Here's how the part is built. I have some questions about the finished solid (model axes, mm). A direction names the side the tool comes from. Coordinates: 2 decimals unless noted, no trailing zeros. Loops run counter-clockwise (first coordinate to the right, second up) from the corner with the lowest first, then second, coordinate; pieces in that order, holes last. Notation, with made-up numbers: M 57,63.25 L 74,63.25 A17 ccw 74,85.25 Z; hole C 87,34.25 d6. An arc over 180 degrees is marked long. Use one line per item in the form item = value. Start each with the question number.
(1) Thinking about a two-plate mould opening in Y: for faces 1 (the flat face through (16, 0, -6)), 2 (the flat face through (1, 10, -6)), 3 (the flat face through (1, 25, -6)), which applies, +Y half, -Y half, draft (parallel to the pull), parting line (faces both ways), or undercut?
(2) Imagine slicing it at D-D, the plane y = -20. Please give me the cut outline in (x, z).
(3) Will these pins go through, and if not, where does the flat tip stop? P1, Ø1, axis at x = 26, y = -4.5, coming from the -Z side; P2, Ø12, axis at x = 0.5, y = -15, coming from the +Z side; P3, Ø1.5, axis at x = 14.5, z = -10.5, coming from the +Y side.
(4) Imagine slicing it at C-C, the plane z = -6. Please give me the cut outline in (x, y), and give its area (3 significant figures).
(5) On a 3-axis mill with a long thin cutter (end or side, diameter ignored), from which of +Z, -Z, +X, -X, +Y, -Y can I reach the whole of each face in a straight line? I mean faces 4 (the flat face through (16, 5, -6)), 5 (the flat face through (6, 20, -6)), 6 (the flat face through (23, -15, -6)). Say none if no direction works.
(6) Imagine slicing it at A-A, the plane y = 22. Please give me the cut outline in (x, z).
(7) Please list where these lines run through material, in increasing order: L1, parallel to X at y = 13.5, z = -10.75; L2, parallel to Y at x = 4, z = -1.5; L3, parallel to Y at x = 11, z = -0.25.
(8) Imagine slicing it at B-B, the plane z = -12.75. Please give me the cut outline in (x, y).
```python
from build123d import *
from build123d.topology import SkipClean

# Parameters (mm, degrees)
SKETCH_3_W          = 32
SKETCH_3_H          = 12
EXTRUDE_3_DEPTH     = 5
SKETCH_4_R          = 5
EXTRUDE_4_DEPTH     = 10
SKETCH_8_R          = 5
EXTRUDE_6_DEPTH     = 5
SKETCH_9_R          = 4.8
CUT_EXTRUDE_2_DEPTH = 0.5
EXTRUDE_START       = 5
SKETCH_36_R         = 5
SKETCH_36_R_2       = 4.98
EXTRUDE_11_DEPTH    = 5
SKETCH_46_W         = 32
SKETCH_46_H         = 12
EXTRUDE_12_DEPTH    = 20
SKETCH_47_W         = 4
SKETCH_47_H         = 25
EXTRUDE_13_DEPTH    = 12
SKETCH_48_W         = 4
SKETCH_48_H         = 25
EXTRUDE_14_DEPTH    = 12
CUT_EXTRUDE_START   = -12
CUT_EXTRUDE_5_DEPTH = 12
SKETCH_50_R         = 6
EXTRUDE_15_DEPTH    = 20
SKETCH_51_R         = 6
EXTRUDE_16_DEPTH    = 20
SKETCH_54_R         = 6
EXTRUDE_17_DEPTH    = 25
SKETCH_55_R         = 6
EXTRUDE_18_DEPTH    = 25
SKETCH_56_R         = 6
CUT_EXTRUDE_6_DEPTH = 10
SKETCH_57_R         = 2.5
EXTRUDE_19_DEPTH    = 10
SKETCH_58_R         = 6
SKETCH_58_R_2       = 2.5
CUT_EXTRUDE_8_DEPTH = 10
EXTRUDE_20_DEPTH    = 2.5
EXTRUDE_21_DEPTH    = 2.5


# Read off the part's stored shape, not the designer's step: the extrude step
with BuildPart() as part:
    # Sketch 3 → Extrude 3 (new body)
    with BuildSketch(Plane(origin=(0, 0, 0), x_dir=(1, 0, 0), z_dir=(0, 1, 0))):
        with Locations((16, 6)):
            Rectangle(SKETCH_3_W, SKETCH_3_H)
    extrude(amount=EXTRUDE_3_DEPTH)

    # Sketch 4 → Extrude 4 (add)
    with BuildSketch(Plane.XZ):
        with Locations(Location((6, -6, 0), (0, 0, 270))):
            Circle(SKETCH_4_R)
        with Locations(Location((26, -6, 0), (0, 0, 270))):
            Circle(SKETCH_4_R)
    extrude(amount=EXTRUDE_4_DEPTH)

    # Sketch 8 → Extrude 6 (add)
    with BuildSketch(Plane.XZ.offset(10)):
        with Locations(Location((6, -6, 0), (0, 0, 270))):
            Circle(SKETCH_8_R)
    extrude(amount=EXTRUDE_6_DEPTH)

    # Sketch 9 → Cut-Extrude 2 (cut)
    with BuildSketch(Plane.XZ.offset(15)):
        with Locations(Location((6, -6, 0), (0, 0, 270))):
            Circle(SKETCH_9_R)
    extrude(amount=-CUT_EXTRUDE_2_DEPTH, mode=Mode.SUBTRACT)



with BuildPart() as body_2:
    # Sketch 14 → Revolve 2 (revolve)
    with BuildSketch(Plane.XY.offset(-6), mode=Mode.PRIVATE) as revolve_2_sk:
        Polygon((1.021282046, -15), (1.021282046, -20), (1.221282046, -15), align=None)
    revolve(revolve_2_sk.sketch.rotate(Axis((6, -15, -6), (0, 1, 0)), 270), axis=Axis((6, -15, -6), (0, 1, 0)))


with BuildPart() as part_1:
    with SkipClean():  # the faces are left unmerged after this step: merging them gives an invalid solid
        add(part.part)

        add(body_2.part)  # Extrude 11 merges body 2
        # Sketch 36 → Extrude 11 (add)
        with BuildSketch(Plane(origin=(0, -20, 0), x_dir=(1, 0, 0), z_dir=(0, 1, 0)).offset(EXTRUDE_START)):
            with Locations(Location((6, 6, 0), (0, 0, 270))):
                Circle(SKETCH_36_R)
            with Locations(Location((6, 6, 0), (0, 0, 90))):
                Circle(SKETCH_36_R_2, mode=Mode.SUBTRACT)
        extrude(amount=-EXTRUDE_11_DEPTH)

    # Sketch 46 → Extrude 12 (add)
    with SkipClean():  # the faces are left unmerged after this step: merging them gives an invalid solid
        with BuildSketch(Plane(origin=(0, 5, 0), x_dir=(1, 0, 0), z_dir=(0, 1, 0))):
            with Locations((16, 6)):
                Rectangle(SKETCH_46_W, SKETCH_46_H)
        extrude(amount=EXTRUDE_12_DEPTH)

    # Sketch 47 → Extrude 13 (add)
    with SkipClean():  # the faces are left unmerged after this step: merging them gives an invalid solid
        with BuildSketch(Plane.XY):
            with Locations((-2, 12.5)):
                Rectangle(SKETCH_47_W, SKETCH_47_H)
        extrude(amount=-EXTRUDE_13_DEPTH)

    # Sketch 48 → Extrude 14 (add)
    with SkipClean():  # the faces are left unmerged after this step: merging them gives an invalid solid
        with BuildSketch(Plane.XY):
            with Locations((34, 12.5)):
                Rectangle(SKETCH_48_W, SKETCH_48_H)
        extrude(amount=-EXTRUDE_14_DEPTH)

    # Cut-Extrude 5 outline → Cut-Extrude 5 (cut)
    with SkipClean():  # the faces are left unmerged after this step: merging them gives an invalid solid
        with BuildSketch(Plane.XY.offset(CUT_EXTRUDE_START)):
            Polygon((26, 25), (6, 25), (6, 15), (1, 15), (1, 5), (31, 5), (31, 15), (26, 15), align=None)
        extrude(amount=CUT_EXTRUDE_5_DEPTH, mode=Mode.SUBTRACT)

    # Sketch 50 → Extrude 15 (add)
    with BuildSketch(Plane.XZ):
        with Locations(Location((6, -6, 0), (0, 0, 270))):
            Circle(SKETCH_50_R)
    extrude(amount=EXTRUDE_15_DEPTH)

    # Sketch 51 → Extrude 16 (add)
    with BuildSketch(Plane.XZ):
        with Locations(Location((26, -6, 0), (0, 0, 270))):
            Circle(SKETCH_51_R)
    extrude(amount=EXTRUDE_16_DEPTH)

    # Sketch 52 → Revolve 3 (revolve)
    with BuildSketch(Plane.XY.offset(-6), mode=Mode.PRIVATE) as revolve_3_sk:
        Polygon((0, -20), (0, -25), (0.2, -20), align=None)
    revolve(revolve_3_sk.sketch.rotate(Axis((6, -20, -6), (0, -1, 0)), 270), axis=Axis((6, -20, -6), (0, -1, 0)))

    # Sketch 53 → Revolve 4 (revolve)
    with BuildSketch(Plane.XY.offset(-6), mode=Mode.PRIVATE) as revolve_4_sk:
        Polygon((20, -20), (20, -25), (20.2, -20), align=None)
    revolve(revolve_4_sk.sketch.rotate(Axis((26, -20, -6), (0, -1, 0)), 270), axis=Axis((26, -20, -6), (0, -1, 0)))

    # Sketch 54 → Extrude 17 (add)
    with BuildSketch(Plane.XZ):
        with Locations(Location((6, -6, 0), (0, 0, 270))):
            Circle(SKETCH_54_R)
    extrude(amount=EXTRUDE_17_DEPTH)

    # Sketch 55 → Extrude 18 (add)
    with BuildSketch(Plane.XZ):
        with Locations(Location((26, -6, 0), (0, 0, 270))):
            Circle(SKETCH_55_R)
    extrude(amount=EXTRUDE_18_DEPTH)

    # Sketch 56 → Cut-Extrude 6 (cut)
    with BuildSketch(Plane.XZ.offset(25)):
        with Locations(Location((6, -6, 0), (0, 0, 270))):
            Circle(SKETCH_56_R)
    extrude(amount=-CUT_EXTRUDE_6_DEPTH, mode=Mode.SUBTRACT)

    # Sketch 57 → Extrude 19 (add)
    with BuildSketch(Plane.XZ.offset(15)):
        with Locations(Location((6, -6, 0), (0, 0, 270))):
            Circle(SKETCH_57_R)
    extrude(amount=EXTRUDE_19_DEPTH)

    # Sketch 58 → Cut-Extrude 8 (cut)
    with BuildSketch(Plane.XZ.offset(25)):
        with Locations(Location((26, -6, 0), (0, 0, 270))):
            Circle(SKETCH_58_R)
        with Locations(Location((26, -6, 0), (0, 0, 270))):
            Circle(SKETCH_58_R_2, mode=Mode.SUBTRACT)
    extrude(amount=-CUT_EXTRUDE_8_DEPTH, mode=Mode.SUBTRACT)

    # Sketch 60 → Extrude 20 (add)
    with BuildSketch(Plane.XY):
        Polygon((-4, 25), (6, 25), (6, 15), (1, 15), (1, 5), (31, 5), (31, 15), (26, 15), (26, 25), (36, 25), (36, 0), (-4, 0), align=None)
    extrude(amount=EXTRUDE_20_DEPTH)

    # Sketch 61 → Extrude 21 (add)
    with BuildSketch(Plane(origin=(0, 0, -12), x_dir=(-1, 0, 0), z_dir=(0, 0, -1))):
        Polygon((-36, 25), (-26, 25), (-26, 15), (-31, 15), (-31, 5), (-1, 5), (-1, 15), (-6, 15), (-6, 25), (4, 25), (4, 0), (-36, 0), align=None)
    extrude(amount=EXTRUDE_21_DEPTH)


solid = part_1.part
```
Answer:
q1.face_1 = -Y half
q1.face_2 = undercut
q1.face_3 = +Y half
q2.outline = C 6,-6 d5; C 26,-6 d5
q3.P1 = -12
q3.P2 = 0
q3.P3 = 5
q4.outline = M -4,0 L 0,0 L 0,-15 L 3.5,-15 L 3.5,-25 L 8.5,-25 L 8.5,-15 L 12,-15 L 12,0 L 20,0 L 20,-15 L 23.5,-15 L 23.5,-25 L 28.5,-25 L 28.5,-15 L 32,-15 L 32,0 L 36,0 L 36,25 L 26,25 L 26,15 L 31,15 L 31,5 L 1,5 L 1,15 L 6,15 L 6,25 L -4,25 Z
q4.area = 960 mm²
q5.face_4 = +Z, -Z
q5.face_5 = +Z, -Z, +Y
q5.face_6 = -Y
q6.outline = M -4,-14.5 L 6,-14.5 L 6,2.5 L -4,2.5 Z; M 26,-14.5 L 36,-14.5 L 36,2.5 L 26,2.5 Z
q7.L1 = -4 to 1, 31 to 36
q7.L2 = -15 to 5, 15 to 25
q7.L3 = 0 to 5
q8.outline = M -4,0 L 36,0 L 36,25 L 26,25 L 26,15 L 31,15 L 31,5 L 1,5 L 1,15 L 6,15 L 6,25 L -4,25 Z
